Check sheet for the modelled part. Datum: model origin and axes. Units: mm. Face numbers are marked on the shaded views. A direction names the side the tool comes from. Coordinates: 2 decimals unless noted, no trailing zeros. Loops run counter-clockwise (first coordinate to the right, second up) from the corner with the lowest first, then second, coordinate; pieces in that order, holes last. Notation, with made-up numbers: (-16, -21.5) - (26, -21.5) arc R15 ccw to (26, -12.5) - close; hole circle Ø9 at (33.25, -7.5). An arc over 180 degrees is marked (long way). Write each question's results on one line, items separated by ' | '. Start each with the question number.
1. Cross-section at B-B (y = 8). Record the cut outline in (x, z), and give its area (3 significant figures).
2. Tool access check on the marked faces 4, 5 and 6. Record the directions out of +Z, -Z, +X, -X, +Y, -Y that give a thin tool (end or side, any length) a straight path to the whole face; none if there is none.
3. Thickness scan on line 1 (X direction, y = 3.75, z = 3.4); line 2 (X direction, y = 5, z = 3.2); line 3 (Z direction, x = 1.5, y = 2.5). Record the ranges inside material, lowest first. Write a range as [from, to].
4. Cross-section at A-A (z = 3.2). Record the cut outline in (x, y).
5. Cross-section at C-C (z = 0.5). Record the cut outline in (x, y), and give its area (3 significant figures).
6. Cross-section at D-D (y = 4.5). Record the cut outline in (x, z), and give its area (3 significant figures).
7. Gauge pin test, flat ends, axial feed: P1, Ø0.8, axis at y = 3.5, z = 3, coming from the +X side; P2, Ø6, axis at x = 1.18, y = 3.62, coming from the +Z side; P3, Ø1.6, axis at y = 3, z = 3.5, coming from the -X side. Record the tip position at first contact, or that the pin passes through.
8. Draft check along X on the marked faces 1, 2 and 3. Enter one of: released by +X, released by -X, zero draft, split by the parting line, or undercut.
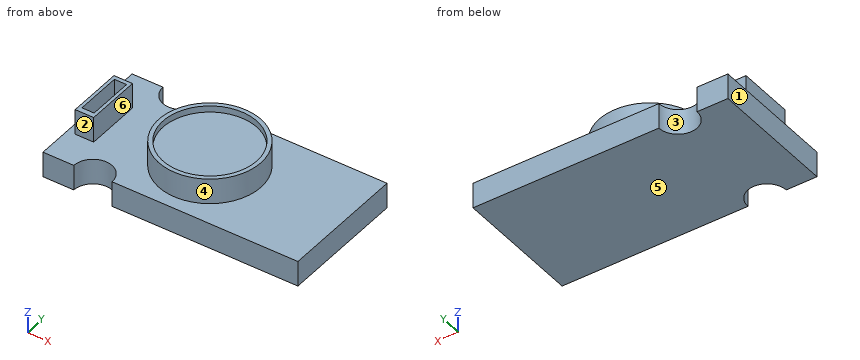
```python
from build123d import *

# Parameters (mm, degrees)
ESQUISSE1_W             = 20
ESQUISSE1_H             = 10
BOSS_EXTRU_1_DEPTH      = 2
ESQUISSE2_R             = 1.5
ENL_V_MAT_EXTRU_1_DEPTH = 2
ESQUISSE3_R             = 4
BOSS_EXTRU_2_DEPTH      = 2
ESQUISSE4_R             = 3.675436607
ENL_V_MAT_EXTRU_2_DEPTH = 0.5
ESQUISSE5_W             = 1.450639668
ESQUISSE5_H             = 4.351919005
BOSS_EXTRU_3_DEPTH      = 2
ESQUISSE6_W             = 0.956804888
ESQUISSE6_H             = 3.642031508
ENL_V_MAT_EXTRU_3_DEPTH = 1.5


with BuildPart() as part:
    # Esquisse1 → Boss.-Extru.1 (new body)
    with BuildSketch(Plane.XY):
        with Locations((1.582964004, 3.620689655)):
            Rectangle(ESQUISSE1_W, ESQUISSE1_H)
    extrude(amount=BOSS_EXTRU_1_DEPTH)

    # Esquisse2 → Enlèv. mat.-Extru.1 (cut)
    with BuildSketch(Plane.XY.offset(2)):
        with Locations((-4.497376734, 8.620689655)):
            Circle(ESQUISSE2_R)
        with Locations((-4.497376734, -1.379310345)):
            Circle(ESQUISSE2_R)
    extrude(amount=-ENL_V_MAT_EXTRU_1_DEPTH, mode=Mode.SUBTRACT)

    # Esquisse3 → Boss.-Extru.2 (add)
    with BuildSketch(Plane.XY.offset(2)):
        with Locations((1.181723245, 3.620689655)):
            Circle(ESQUISSE3_R)
    extrude(amount=BOSS_EXTRU_2_DEPTH)

    # Esquisse4 → Enlèv. mat.-Extru.2 (cut)
    with BuildSketch(Plane.XY.offset(4)):
        with Locations((1.181723245, 3.620689655)):
            Circle(ESQUISSE4_R)
    extrude(amount=-ENL_V_MAT_EXTRU_2_DEPTH, mode=Mode.SUBTRACT)

    # Esquisse5 → Boss.-Extru.3 (add)
    with BuildSketch(Plane.XY.offset(2)):
        with Locations((-7.074576996, 3.528095633)):
            Rectangle(ESQUISSE5_W, ESQUISSE5_H)
    extrude(amount=BOSS_EXTRU_3_DEPTH)

    # Esquisse6 → Enlèv. mat.-Extru.3 (cut)
    with BuildSketch(Plane.XY.offset(4)):
        with Locations((-7.074576996, 3.574392644)):
            Rectangle(ESQUISSE6_W, ESQUISSE6_H)
    extrude(amount=-ENL_V_MAT_EXTRU_3_DEPTH, mode=Mode.SUBTRACT)


solid = part.part
```
Established:
1) outline: (-8.42, 0) - (-5.86, 0) - (-5.86, 2) - (-8.42, 2) - close; (-3.13, 0) - (11.58, 0) - (11.58, 2) - (-3.13, 2) - close | area: 34.5 mm^2
2) face 4: +Z | face 5: -Z, +X, -X, +Y, -Y | face 6: +Z, +Y, -Y
3) line 1: [-7.8, -7.55], [-6.6, -6.35], [-2.82, 5.18] | line 2: [-7.8, -7.55], [-6.6, -6.35], [-2.57, 4.94] | line 3: [0, 3.5]
4) outline: (-7.8, 1.35) - (-6.35, 1.35) - (-6.35, 5.7) - (-7.8, 5.7) - close; circle Ø8 at (1.18, 3.62); hole (-7.55, 1.75) - (-6.6, 1.75) - (-6.6, 5.4) - (-7.55, 5.4) - close
5) outline: (-8.42, -1.38) - (-6, -1.38) arc R1.5 cw to (-3, -1.38) - (11.58, -1.38) - (11.58, 8.62) - (-3, 8.62) arc R1.5 cw to (-6, 8.62) - (-8.42, 8.62) - close | area: 193 mm^2
6) outline: (-8.42, 0) - (11.58, 0) - (11.58, 2) - (5.08, 2) - (5.08, 4) - (4.75, 4) - (4.75, 3.5) - (-2.39, 3.5) - (-2.39, 4) - (-2.72, 4) - (-2.72, 2) - (-6.35, 2) - (-6.35, 4) - (-6.6, 4) - (-6.6, 2.5) - (-7.55, 2.5) - (-7.55, 4) - (-7.8, 4) - (-7.8, 2) - (-8.42, 2) - close | area: 53.5 mm^2
7) P1: x = 5.18 | P2: z = 3.5 | P3: x = -7.8
8) face 1: released by -X | face 2: zero draft | face 3: undercut
